Work out the finished part from the listing and answer in its coordinate system (mm). A direction names the side the tool comes from. Round coordinates to 2 decimals unless told otherwise and drop trailing zeros. Loops run counter-clockwise (first coordinate to the right, second up) from the corner with the lowest first, then second, coordinate; pieces in that order, holes last. Notation, with made-up numbers: (4.5, 31.5) -> (41.5, 31.5) arc R5 cw to (41.5, 39.5) -> close; hole circle Ø1 at (11, 41.5). An arc over 180 degrees is marked (long way). Use one line per item in the form item = value.
Autodesk Inventor part; units mm, degrees
ref_plane "YZ Plane" through (0, 0, 0) normal (1, 0, 0) x (0, 1, 0)
ref_plane "XZ Plane" through (0, 0, 0) normal (0, 1, 0) x (-1, 0, 0)
ref_plane "XY Plane" through (0, 0, 0) normal (0, 0, 1) x (1, 0, 0)
sketch "Sketch1" plane through (0, 0, 0) normal (0, 0, 1) x (1, 0, 0)
  arc A0 (0.1634, -121.6592) -> (226.5563, -100.6675) centre (0.1634, 1109.6463) ccw
  arc A1 (0.1634, -136.6592) -> (216.7225, -117.7003) centre (0.1634, 1109.6463) ccw
  line L0 (226.5563, -100.6675) -> (216.7225, -117.7003)
  line L1 (226.5563, -100.6675) -> (246.2241, -100.6675) construction
  line L2 (0.1634, -136.6592) -> (0.1634, -109.1839)
  arc A2 (-226.2295, -100.6675) -> (0.1634, -121.6592) centre (0.1634, 1109.6463) ccw
  arc A3 (-216.3956, -117.7003) -> (0.1634, -136.6592) centre (0.1634, 1109.6463) ccw
  line L3 (-226.2295, -100.6675) -> (-216.3956, -117.7003)
  point P0 (0, 0)
  point P1 (171.9535, -124.7627)
  dimension "d0" = 15
  dimension "d1" = 120
extrude "Extrusion1" add sketch "Sketch1" along normal blind 30
fillet "Fillet1" radius 3 12 edges at (-113.5186, -116.4001, 30) (108.8571, -131.9105, 30) (221.6394, -109.1839, 30) (216.7225, -117.7003, 15) (226.5563, -100.6675, 15) (221.6394, -109.1839, 0) (113.8455, -116.4001, 0) (-221.3125, -109.1839, 30) (-226.2295, -100.6675, 15) (108.8571, -131.9105, 0) (-216.3956, -117.7003, 15) (-221.3125, -109.1839, 0)
sketch "Sketch2" plane through (0, 0, 0) normal (0, 1, 0) x (-1, 0, 0)
  line L0 (0, 0) -> (0, 15)
  circle A0 centre (0, 15) radius 5
  dimension "d5" = 15
  dimension "d6" = 10
extrude "Extrusion2" cut sketch "Sketch2" against normal blind 300
properties part number "LEAF 5" material "Steel, Carbon"
(1) Find section A-A, the plane z = 15. Write down the section's boundary in (x, y), then the cut area to 3 significant figures.
Completed:
outline = (-222.98, -106.3) -> (-217.1, -116.49) arc R3 ccw to (-215.02, -117.94) arc R1246.3 ccw to (-5, -136.65) -> (-5, -121.65) arc R1231.31 cw to (-219.85, -101.84) arc R3 ccw to start; (5, -136.65) arc R1246.31 ccw to (215.34, -117.94) arc R3 ccw to (217.42, -116.49) -> (223.31, -106.3) arc R3 ccw to (220.17, -101.84) arc R1231.31 cw to (5, -121.65) -> close
area = 6,510 mm2
(2) Given P1, Ø12, axis at y = -120, z = 17.5, coming from the -X side, flat-ended and moving along its own axis, determine where the tip first touches the part or whether it passes through.
Completed:
P1 = -218.53
(3) For faces 1 (the cylindrical face through (-108.744, -116.833, 14.832)), 2 (the cylindrical face through (-106.32, -132.1, 14.83)), determine the directions among +Z, -Z, +X, -X, +Y, -Y from which every point of the face is accessible in a straight line to the end or side of a thin tool.
Completed:
face_1 = +Z, -Z, +Y
face_2 = +Z, -Z, -X, -Y
(4) For a pull along X with two mould halves and no side action, classify faces 3 (the cylindrical face through (112.155, -116.556, 14.832)), 4 (the cylindrical face through (219.542, -111.012, 0.855)), 5 (the cylindrical face through (-219.256, -111.036, 0.902)) as +X half, -X half, draft (parallel to the pull), parting line (faces both ways), or undercut.
Completed:
face_3 = undercut
face_4 = +X half
face_5 = -X half
(5) Consider L1, parallel to Z at x = 0, y = -131.5; L2, parallel to Z at x = -201, y = -108; L3, parallel to Y at x = 170, z = 16. Determine where each line is inside the solid, lowest interval first.
Completed:
L1 = 0 to 10, 20 to 30
L2 = 0 to 30
L3 = -125.03 to -109.89
